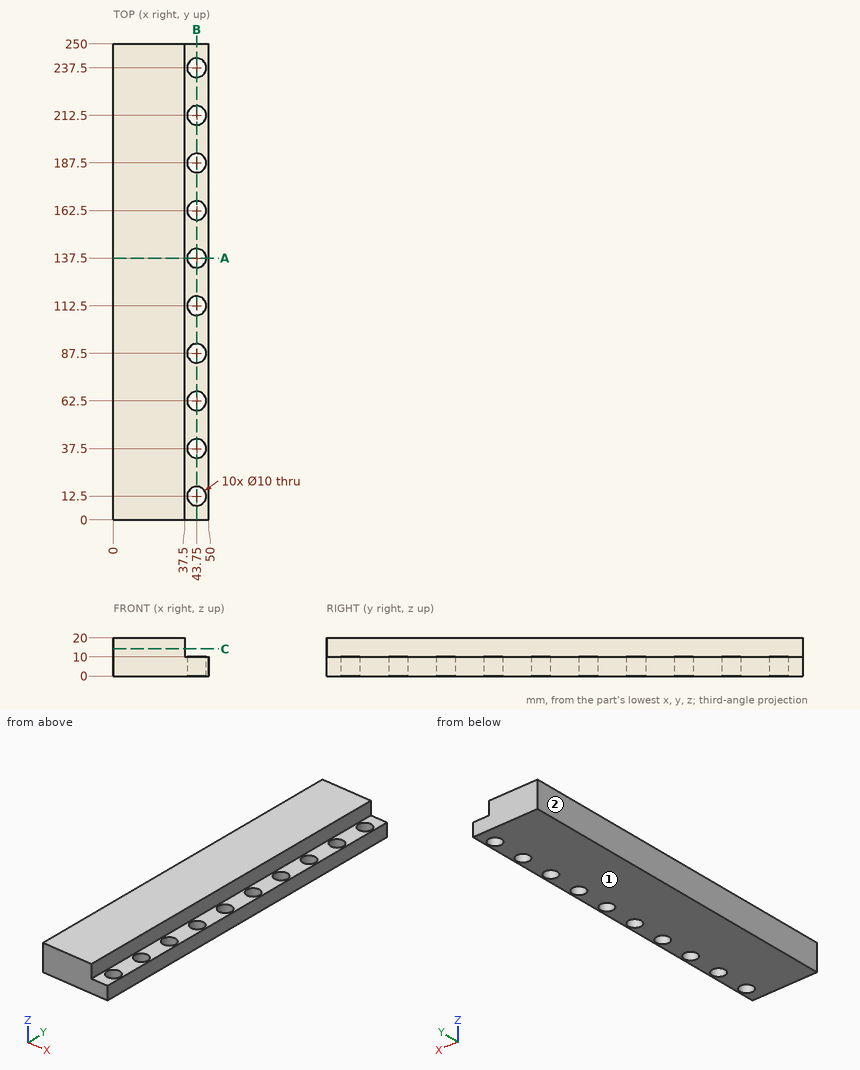
Verification items for this drawing (mm, ordinates from the low corner). Coordinates: 2 decimals unless noted, no trailing zeros. Write each loop counter-clockwise with the first axis right and the second up, starting at its lowest first coordinate (ties: lowest second). Pieces come first, ordered by that corner, then holes. Notation, with made-up numbers: (30, 16) -> (57, 16) arc R27 cw to (57, 40) -> close; hole circle Ø2 at (5, 62). An arc over 180 degrees is marked (long way). One line per item, written item: value. Start each with the question number.
Q1. Thickness scan on L1, parallel to X at y = 139, z = 18; L2, parallel to Z at x = 39.5, y = 84; L3, parallel to X at y = 217, z = 7. Record the ranges inside material, lowest first. Write a range as from..to.
Q2. Cross-section at A-A on y = 137.5. Enter the section's corners in (x, z).
Q3. Go/stop test with a flat-tipped pin: P1, Ø9, axis at x = 43.75, y = 237.5, coming from the -Z side. Record where the tip stops, or that it passes through.
Q4. Cross-section at B-B on x = 43.75. State how many separate pieces and enclosed holes the cut face has, and give its area (3 significant figures).
Q5. Mould release check, pull along X, two halves, no side actions. Record for the marked faces 1 and 2: pulls with the +X half, pulls with the -X half, needs draft (parallel to the pull), parting line crosses it, or undercut.
Q6. Cross-section at C-C on z = 14.25. Enter the section's corners in (x, y), and give its area (4 significant figures).
Checked values:
1. L1: x = 0..37.5
1. L2: z = 0..10
1. L3: x = 0..41.57, 45.93..50
2. outline: (0, 0) -> (38.75, 0) -> (38.75, 10) -> (37.5, 10) -> (37.5, 20) -> (0, 20) -> close; (48.75, 0) -> (50, 0) -> (50, 10) -> (48.75, 10) -> close
3. P1: passes through
4. separate pieces: 11
4. enclosed holes: 0
4. area: 1,500 mm²
5. face 1: needs draft
5. face 2: pulls with the -X half
6. outline: (0, 0) -> (37.5, 0) -> (37.5, 250) -> (0, 250) -> close
6. area: 9,375 mm²
